```python
from build123d import *

# Parameters (mm, degrees)
SKETCH_1_W          = 60
SKETCH_1_H          = 32.5
EXTRUDE_1_DEPTH     = 25
SKETCH_2_W          = 34
SKETCH_2_H          = 34
EXTRUDE_2_DEPTH     = 25
SKETCH_2_2_W        = 34
SKETCH_2_2_H        = 34
EXTRUDE_3_DEPTH     = 42
SKETCH_3_W          = 38
SKETCH_3_H          = 34
CUT_EXTRUDE_1_DEPTH = 91.65870063
SKETCH_4_R          = 2.75
CUT_EXTRUDE_2_DEPTH = 76.802374633
SKETCH_5_R          = 2.75
CUT_EXTRUDE_3_DEPTH = 75.143442057
SKETCH_6_R          = 5
CUT_EXTRUDE_4_DEPTH = 7.5
SKETCH_7_R          = 5
CUT_EXTRUDE_5_DEPTH = 78.21398837
SKETCH_8_R          = 12
CUT_EXTRUDE_6_DEPTH = 4


with BuildPart() as part:
    # Эскиз1 → Бобышка-Вытянуть1 (new body)
    with BuildSketch(Plane.XY):
        with Locations((30, 16.25)):
            Rectangle(SKETCH_1_W, SKETCH_1_H)
    extrude(amount=EXTRUDE_1_DEPTH)

    # Эскиз2 → Бобышка-Вытянуть2 (add)
    with BuildSketch(Plane.XY.offset(25)):
        with Locations((30, 22)):
            Rectangle(SKETCH_2_W, SKETCH_2_H)
    extrude(amount=-EXTRUDE_2_DEPTH)

    # Эскиз2<2> → Бобышка-Вытянуть3 (add)
    with BuildSketch(Plane.XY.offset(25)):
        with Locations((30, 22)):
            Rectangle(SKETCH_2_2_W, SKETCH_2_2_H)
    extrude(amount=EXTRUDE_3_DEPTH)

    # Эскиз3 → Вырез-Вытянуть1 (cut, through all)
    with BuildSketch(Plane(origin=(47, 0, 0), x_dir=(0, 0, -1), z_dir=(1, 0, 0))):
        with Locations((-48, 22)):
            Rectangle(SKETCH_3_W, SKETCH_3_H)
    extrude(amount=-CUT_EXTRUDE_1_DEPTH, mode=Mode.SUBTRACT)

    # Эскиз4 → Вырез-Вытянуть2 (cut, through all)
    with BuildSketch(Plane.XY.offset(25)):
        with Locations((7, 22)):
            Circle(SKETCH_4_R)
        with Locations((7, 7)):
            Circle(SKETCH_4_R)
        with Locations((53, 7)):
            Circle(SKETCH_4_R)
        with Locations((53, 22)):
            Circle(SKETCH_4_R)
    extrude(amount=-CUT_EXTRUDE_2_DEPTH, mode=Mode.SUBTRACT)

    # Эскиз5 → Вырез-Вытянуть3 (cut, through all)
    with BuildSketch(Plane(origin=(0, 32.5, 0), x_dir=(1, 0, 0), z_dir=(0, 1, 0))):
        with Locations(Location((7, -19, 0), (0, 0, 180))):
            Circle(SKETCH_5_R)
        with Locations(Location((7, -6, 0), (0, 0, 180))):
            Circle(SKETCH_5_R)
        with Locations(Location((53, -6, 0), (0, 0, 180))):
            Circle(SKETCH_5_R)
        with Locations(Location((53, -19, 0), (0, 0, 180))):
            Circle(SKETCH_5_R)
    extrude(amount=-CUT_EXTRUDE_3_DEPTH, mode=Mode.SUBTRACT)

    # Эскиз6 → Вырез-Вытянуть4 (cut)
    with BuildSketch(Plane(origin=(0, 32.5, 0), x_dir=(1, 0, 0), z_dir=(0, 1, 0))):
        with Locations(Location((7, -6, 0), (0, 0, 270))):
            Circle(SKETCH_6_R)
        with Locations(Location((7, -19, 0), (0, 0, 270))):
            Circle(SKETCH_6_R)
        with Locations(Location((53, -19, 0), (0, 0, 270))):
            Circle(SKETCH_6_R)
        with Locations(Location((53, -6, 0), (0, 0, 270))):
            Circle(SKETCH_6_R)
    extrude(amount=-CUT_EXTRUDE_4_DEPTH, mode=Mode.SUBTRACT)

    # Эскиз7 → Вырез-Вытянуть5 (cut, through all)
    with BuildSketch(Plane.XY.offset(29)):
        with Locations((30, 22)):
            Circle(SKETCH_7_R)
    extrude(amount=-CUT_EXTRUDE_5_DEPTH, mode=Mode.SUBTRACT)

    # Эскиз8 → Вырез-Вытянуть6 (cut)
    with BuildSketch(Plane.XY.offset(29)):
        with Locations((30, 22)):
            Circle(SKETCH_8_R)
    extrude(amount=-CUT_EXTRUDE_6_DEPTH, mode=Mode.SUBTRACT)


solid = part.part
```
Read the model definition and answer for the solid it produces. Units are mm, in the model's axes. A direction names the side the tool comes from. Give positions to 0.01 mm unless a question says otherwise; leave off trailing zeros. Write each loop counter-clockwise with the first axis right and the second up, starting at its lowest first coordinate (ties: lowest second). Pieces come first, ordered by that corner, then holes. Notation, with made-up numbers: (-18.5, 64) - (16.5, 64) arc R16 cw to (16.5, 79) - close; hole circle Ø8 at (54, 60). An arc over 180 degrees is marked (long way). Write item = value, one per line. Start each with the question number.
Item 1: Find section D-D (x = 45). Give the vertices of the cut face in (y, z).
Item 2: Find section C-C (y = 14). Give the vertices of the cut face in (x, z).
Item 3: Find section B-B (z = 26). Give the vertices of the cut face in (x, y), then the cut area to 3 significant figures.
Item 4: A tool of negligible diameter and unlimited length cuts with its end or side. For faces 1 (the flat face through (35.2, 22.2, 25)), 2 (the flat face through (53, 32.5, 12)), 3 (the flat face through (50.8, 25, 8.2)), from which of +Z, -Z, +X, -X, +Y, -Y can it reach the whole face along a straight path? Write none if from no direction.
Item 5: Find the intervals of material crossed by probe 1 along X at (y, z) = (2.5, 6); probe 2 along Y at (x, z) = (4.5, 21.5); probe 3 along Z at (x, y) = (5.5, 12), in increasing order. Write a range as [from, to].
Item 6: The mould has two halves that part along Z. Classify faces 4 (the flat face through (30, 15, 0)), 5 (the cylindrical face through (11.957, 28.803, 18.349)), 6 (the cylindrical face through (4.973, 23.859, 2.375)), 7 (the flat face through (50.8, 25, 21.2)): +Z half, -Z half, draft (parallel to the pull), parting line (faces both ways), or undercut.
Item 7: Find section A-A (x = 30). Give the vertices of the cut face in (y, z), then the cut area to 3 significant figures.
Item 8: This flat-tipped pin is pushed along its axis until it touches: P1, Ø3, axis at x = 54.5, z = 21, coming from the +Y side. Where does it stop, or does it pass through?
Response:
q1.outline = (0, 0) - (39, 0) - (39, 29) - (5, 29) - (5, 25) - (0, 25) - close
q2.outline = (0, 0) - (60, 0) - (60, 25) - (47, 25) - (47, 29) - (38.94, 29) - (38.94, 25) - (21.06, 25) - (21.06, 29) - (13, 29) - (13, 25) - (0, 25) - close; hole circle Ø5.5 at (7, 6); hole circle Ø5.5 at (7, 19); hole circle Ø5.5 at (53, 6); hole circle Ø5.5 at (53, 19)
q3.outline = (13, 5) - (47, 5) - (47, 39) - (13, 39) - close; hole circle Ø24 at (30, 22)
q3.area = 704 mm²
q4.face_1 = +Z
q4.face_2 = +Z, -Z, +X, +Y
q4.face_3 = +Y
q5.probe_1 = [0, 4.25], [9.75, 50.25], [55.75, 60]
q5.probe_2 = [0, 5.85], [8.15, 20.85], [23.15, 25]
q5.probe_3 = [0, 3.7], [8.3, 16.7], [21.3, 25]
q6.face_4 = -Z half
q6.face_5 = undercut
q6.face_6 = draft
q6.face_7 = undercut
q7.outline = (0, 0) - (17, 0) - (17, 25) - (10, 25) - (10, 29) - (5, 29) - (5, 25) - (0, 25) - close; (27, 0) - (39, 0) - (39, 29) - (34, 29) - (34, 25) - (27, 25) - close
q7.area = 765 mm²
q8.P1 = 25
